Build history of the part. All positions in model axes, mm. A direction names the side the tool comes from. Give positions to 0.01 mm unless a question says otherwise; leave off trailing zeros. Write each loop counter-clockwise with the first axis right and the second up, starting at its lowest first coordinate (ties: lowest second). Pieces come first, ordered by that corner, then holes. Notation, with made-up numbers: (31, 29.5) - (85, 29.5) arc R16 ccw to (85, 47.5) - close; hole circle Ø2 at (6.25, 38). An arc over 180 degrees is marked (long way). Use one line per item in the form item = value. Start each with the question number.
from build123d import *

# Parameters (mm, degrees)
F0_W     = 112
F0_H     = 66
F1_DEPTH = 25
F2_W     = 108
F2_H     = 62
F3_DEPTH = 23
F5_DEPTH = 3.5
F6_W     = 1.2
F6_H     = 5
F6_H_2   = 1.5
F7_DEPTH = 5


with BuildPart() as f1:
    # F0 (on Top) → F1 (new body)
    with BuildSketch(Plane.XY):
        with Locations((7.001376, -11.34)):
            Rectangle(F0_W, F0_H)
    extrude(amount=F1_DEPTH)

    # F2 (on face) → F3 (cut)
    with BuildSketch(Plane.XY.offset(25)):
        with Locations((7.001376, -11.34)):
            Rectangle(F2_W, F2_H)
    extrude(amount=-F3_DEPTH, mode=Mode.SUBTRACT)

    # F4 (on face) → F5 (join)
    with BuildSketch(Plane.XY.offset(2)):
        Polygon((-28.198624, 7.16), (-28.198624, 18.36), (55.101376, 18.36), (55.101376, -41.04), (-28.198624, -41.04), (-28.198624, -28.84), (-29.498624, -28.84), (-29.498624, -42.34), (56.401376, -42.34), (56.401376, 19.66), (-29.498624, 19.66), (-29.498624, 7.16), align=None)
    extrude(amount=F5_DEPTH)

    # F6 (on face) → F7 (join)
    with BuildSketch(Plane.XY.offset(2)):
        with Locations((57.001376, 17.16)):
            Rectangle(F6_W, F6_H)
        with Locations((-30.098624, -41.59)):
            Rectangle(F6_W, F6_H_2)
        with Locations((57.001376, -41.59)):
            Rectangle(F6_W, F6_H_2)
        with Locations((-30.098624, 17.16)):
            Rectangle(F6_W, F6_H)
    extrude(amount=F7_DEPTH)


solid = f1.part
(1) Wall check: line 1 (X direction, y = 3.5, z = 3.5); line 2 (X direction, y = -40.5, z = 3.75); line 3 (X direction, y = -14, z = 20.25). Give the ranges that are in metal, low to high. Write a range as from..to.
(2) Two-plate mould, pull along Y, no slides. Class faces 3 (the flat face through (6, -11, 0)), 4 (the flat face through (55.101, -11, 4)), 5 (the flat face through (6, -44.34, 12)): +Y half, -Y half, draft (parallel to the pull), parting line (faces both ways), or undercut.
(3) Pin check, flat tips, straight feed: pin 1 Ø2.5 at (x, y) = (59, -5.5) entering from +Z; pin 2 Ø1 at (x, y) = (57, -41.5) entering from +Z. Stop position of each tip, or through.
(4) Cut at D-D, the plane y = -32. Give the cut face in (x, z).
(5) Cut at A-A, the plane z = 21.5. Give the cut face in (x, y).
(6) Cut at C-C, the plane x = 42.5. Give the cut face in (y, z).
(7) Cut at B-B, the plane y = -5. Give the cut face in (x, z), then the cut area to 3 significant figures.
(8) Which spindle directions (+Z, -Z, +X, -X, +Y, -Y) get a long thin tool onto all of the face, cutting with end or side? Do faces 1 (the flat face through (63.001, -12, 12)), 2 (the flat face through (-30.699, 17, 4)). Say none if no direction does.
Solution:
q1.line_1 = -49..-47, 55.1..56.4, 61..63
q1.line_2 = -49..-47, -29.5..-28.2, 55.1..56.4, 61..63
q1.line_3 = -49..-47, 61..63
q2.face_3 = draft
q2.face_4 = undercut
q2.face_5 = -Y half
q3.pin_1 = 2
q3.pin_2 = 7
q4.outline = (-49, 0) - (63, 0) - (63, 25) - (61, 25) - (61, 2) - (56.4, 2) - (56.4, 5.5) - (55.1, 5.5) - (55.1, 2) - (-28.2, 2) - (-28.2, 5.5) - (-29.5, 5.5) - (-29.5, 2) - (-47, 2) - (-47, 25) - (-49, 25) - close
q5.outline = (-49, -44.34) - (63, -44.34) - (63, 21.66) - (-49, 21.66) - close; hole (-47, -42.34) - (61, -42.34) - (61, 19.66) - (-47, 19.66) - close
q6.outline = (-44.34, 0) - (21.66, 0) - (21.66, 25) - (19.66, 25) - (19.66, 5.5) - (18.36, 5.5) - (18.36, 2) - (-41.04, 2) - (-41.04, 5.5) - (-42.34, 5.5) - (-42.34, 25) - (-44.34, 25) - close
q7.outline = (-49, 0) - (63, 0) - (63, 25) - (61, 25) - (61, 2) - (56.4, 2) - (56.4, 5.5) - (55.1, 5.5) - (55.1, 2) - (-47, 2) - (-47, 25) - (-49, 25) - close
q7.area = 321 mm2
q8.face_1 = +Z, -Z, +X, +Y, -Y
q8.face_2 = +Z
